Can you work these out from the model? Positions are in its coordinate system, mm. A direction names the side the tool comes from. Round coordinates to 2 decimals unless told otherwise and drop trailing zeros. Order: outer loops, then holes, each group sorted by start corner. A loop starts at its lowest first (then second) coordinate and runs counter-clockwise, first axis right, second up. Notation, with made-up numbers: (-6.75, 76) - (16.25, 76) arc R34 cw to (16.25, 107) - close; hole circle Ø9 at (-36, 11). An arc over 180 degrees is marked (long way). Write item = value, one per line.
from build123d import *

# Parameters (mm, degrees)
SKETCH_1_R      = 70
SKETCH_1_R_2    = 14.438127561
EXTRUDE_1_DEPTH = 40
SKETCH_2_R      = 14.438127561
SKETCH_2_R_2    = 10
EXTRUDE_2_DEPTH = 40
FILLET_1_R      = 2


with BuildPart() as part:
    # 草图1 → 凸台-拉伸1 (new body)
    with BuildSketch(Plane.XY.offset(70.26)):
        with Locations((-553.234692624, 615.626439551)):
            Circle(SKETCH_1_R)
        with Locations((-553.234692624, 615.626439551)):
            Circle(SKETCH_1_R_2, mode=Mode.SUBTRACT)
    extrude(amount=-EXTRUDE_1_DEPTH)

    # 草图2 → 凸台-拉伸2 (add)
    with BuildSketch(Plane.XY.offset(70.26)):
        with Locations((-553.234692624, 615.626439551)):
            Circle(SKETCH_2_R)
        with Locations((-553.234692624, 615.626439551)):
            Circle(SKETCH_2_R_2, mode=Mode.SUBTRACT)
    extrude(amount=-EXTRUDE_2_DEPTH)

    # 草图4 → 切除-旋转1 (revolve, cut)
    with BuildSketch(Plane(origin=(0, 615.626439551, 0), x_dir=(1, 0, 0), z_dir=(0, 1, 0))):
        with BuildLine():
            Line((-493.814063129, -48.26), (-493.814063129, -52.26))
            ThreePointArc((-493.814063129, -52.26), (-490.181232126, -58.451059372), (-483.234692624, -60.26))
            Line((-483.234692624, -60.26), (-483.234692624, -40.26))
            ThreePointArc((-483.234692624, -40.26), (-490.181232126, -42.068940628), (-493.814063129, -48.26))
        make_face()
    revolve(axis=Axis((-553.234692624, 615.626439551, 70.26), (0, 0, -1)), mode=Mode.SUBTRACT)

    # 圆角1
    fillet_1_edges = [part.edges().sort_by_distance(p)[0] for p in [
        (-623.234692624, 615.626439551, 70.26),
        (-623.234692624, 615.626439551, 30.26),
    ]]
    fillet(fillet_1_edges, radius=FILLET_1_R)


solid = part.part
(1) On a 3-axis mill with a long thin cutter (end or side, diameter ignored), from which of +Z, -Z, +X, -X, +Y, -Y can I reach the whole of each face in a straight line? I mean faces 1 (the face through (-597.03, 575.467, 50.288)), 2 (the face through (-554, 601, 70.26)). Say none if no direction works.
Computed:
face_1 = none
face_2 = +Z, +X, -X, +Y, -Y
(2) Thinking about a two-plate mould opening in Y: for faces 3 (the face through (-554, 601, 30.26)), 4 (the face through (-548.62, 606.755, 50.54)), 5 (the face through (-604.828, 662.936, 36.316)), which applies, +Y half, -Y half, draft (parallel to the pull), parting line (faces both ways), or undercut?
Computed:
face_3 = draft
face_4 = undercut
face_5 = parting line
(3) If I drill on line 1 (Z direction, x = -595, y = 667); line 2 (Z direction, x = -488.5, y = 633); line 3 (Y direction, x = -551, z = 49), over which ranges is the centre line in solid material (lowest first)? Write a range as from..to.
Computed:
line_1 = 30.26..40.51, 60.01..70.26
line_2 = 30.26..40.32, 60.2..70.26
line_3 = 556.25..605.88, 625.37..675.01
(4) If we section it at A-A (z = 38.5): Write out the boundary of the cut face in (x, y).
Computed:
outline = circle Ø140 at (-553.23, 615.63); hole circle Ø20 at (-553.23, 615.63)
(5) Will these pins go through, and if not, where does the flat tip stop? P1, Ø6, axis at y = 597.5, z = 61.5, coming from the -X side; P2, Ø1, axis at y = 585, z = 65, coming from the +X side; P3, Ø10, axis at x = -502.5, z = 63, coming from the +Y side.
Computed:
P1 = -621.58
P2 = -490.05
P3 = 668.62
